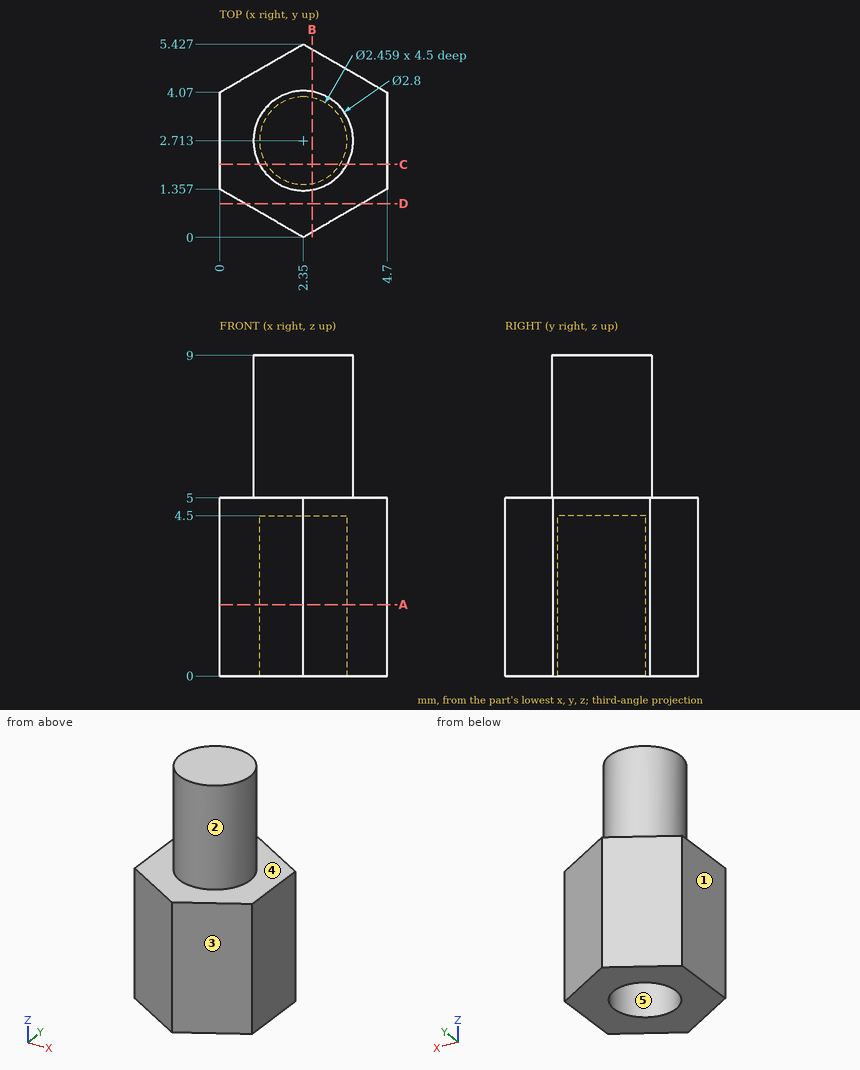
Input: dimensioned drawing with shaded views. Units: mm. Origin: part minimum x, y, z. A direction names the side the tool comes from. Coordinates: 2 decimals unless noted, no trailing zeros. Write each loop counter-clockwise with the first axis right and the second up, starting at its lowest first coordinate (ties: lowest second). Pieces come first, ordered by that corner, then holes. Notation, with made-up numbers: M 78,-2 L 135,-2 A4 ccw 135,4 Z; hole C 15,57.5 d7. An arc over 180 degrees is marked long. Use one line per item in the form item = value.
Q1. Material intervals for probe 1 along X at (y, z) = (3.1, 1.5); probe 2 along X at (y, z) = (1.95, 2.25) (1 decimal); probe 3 along Z at (x, y) = (2.8, 4.45), sorted ascending. Write a range as from..to.
Answer below:
probe_1 = 0..1.18, 3.52..4.7
probe_2 = 0..1.4, 3.3..4.7
probe_3 = 0..5
Q2. Set-up query: the marked faces 1 and 2. Return all of +Z, -Z, +X, -X, +Y, -Y with unobstructed straight access to the full face (end or side cutting, diameter ignored); none if empty.
Answer below:
face_1 = +Z, -Z, -X, +Y, -Y
face_2 = +Z
Q3. Section D-D (y = 0.95). Return loops of the section in (x, z) (1 decimal).
Answer below:
outline = M 0.7,0 L 4,0 L 4,5 L 0.7,5 Z
Q4. Section B-B (x = 2.6). Return loops of the section in (y, z) (1 decimal).
Answer below:
outline = M 0.1,0 L 1.5,0 L 1.5,4.5 L 3.9,4.5 L 3.9,0 L 5.3,0 L 5.3,5 L 4.1,5 L 4.1,9 L 1.3,9 L 1.3,5 L 0.1,5 Z
Q5. Draft query along X for the marked faces 3, 4 and 5. Return one class per face: released by +X, released by -X, zero draft, split by the parting line, or undercut.
Answer below:
face_3 = released by +X
face_4 = zero draft
face_5 = undercut
Q6. Section C-C (y = 2.05). Return loops of the section in (x, z) (1 decimal).
Answer below:
outline = M 0,0 L 1.3,0 L 1.3,4.5 L 3.4,4.5 L 3.4,0 L 4.7,0 L 4.7,5 L 3.6,5 L 3.6,9 L 1.1,9 L 1.1,5 L 0,5 Z
Q7. Section A-A (z = 2). Return loops of the section in (x, y).
Answer below:
outline = M 0,1.36 L 2.35,0 L 4.7,1.36 L 4.7,4.07 L 2.35,5.43 L 0,4.07 Z; hole C 2.35,2.71 d2.46
